Work out the finished part from the listing and answer in its coordinate system (mm). Round coordinates to 2 decimals unless told otherwise and drop trailing zeros. Order: outer loops, then holes, each group sorted by start corner. A loop starts at its lowest first (then second) coordinate and runs counter-clockwise, first axis right, second up. Notation, with made-up numbers: (24.5, 55) - (51.5, 55) arc R36 ccw to (51.5, 90) - close; hole circle Ø3 at (20, 75.25). An arc over 180 degrees is marked (long way). Use one line per item in the form item = value. Start each with the question number.
Q1. The part is cut by section D-D on x = 12.5. Determine the outline of the cut face in (y, z), plus the area to 3 significant figures.
Q2. The part is cut by section C-C on x = -74.5. Determine the outline of the cut face in (y, z), plus the area to 3 significant figures.
Q3. Given P1, Ø3, axis at y = -37.5, z = 2.5, coming from the +X side; P2, Ø6, axis at x = -55, z = 4.5, coming from the +Y side; P3, Ø2, axis at x = 41, z = 2.5, coming from the +Y side, each flat-ended and moving along its own axis, determine where each tip first touches the part or whether it passes through.
Q4. The part is cut by section A-A on z = 8.25. Determine the outline of the cut face in (x, y).
Q5. Find the intervals of material crossed by line 1 (X direction, y = 34, z = 1.25); line 2 (Y direction, x = 45.5, z = 9.75); line 3 (X direction, y = -78, z = 5.25), in increasing order. Write a range as [from, to].
Q6. The part is cut by section B-B on y = 0. Determine the outline of the cut face in (x, z).
from build123d import *

# Parameters (mm, degrees)
SKETCH2_R           = 40
BOSS_EXTRUDE1_DEPTH = 10


with BuildPart() as part:
    # Sketch2 → Boss-Extrude1 (new body)
    with BuildSketch(Plane.XY):
        with BuildLine():
            Line((-100, -40), (-100, -30))
            ThreePointArc((-100, -30), (-70, 0), (-100, 30))
            Line((-100, 30), (-100, 40))
            ThreePointArc((-100, 40), (-84.220237409, 36.755939555), (-71, 27.549954628))
            ThreePointArc((-71, 27.549954628), (-55.218260111, 21.366045629), (-40.357142857, 29.51780853))
            ThreePointArc((-40.357142857, 29.51780853), (-23.282031855, 44.248694813), (-1.47081146, 49.978362455))
            ThreePointArc((-1.47081146, 49.978362455), (15.390674553, 60.197087002), (15.293909304, 79.913138291))
            ThreePointArc((15.293909304, 79.913138291), (11.346128086, 89.510287366), (10, 99.8))
            Line((10, 99.8), (20, 99.8))
            ThreePointArc((20, 99.8), (50, 69.8), (80, 99.8))
            Line((80, 99.8), (90, 99.8))
            ThreePointArc((90, 99.8), (79.950139168, 73.286057181), (54.85054181, 60.095186134))
            ThreePointArc((54.85054181, 60.095186134), (39.000828287, 48.368352667), (40.911294797, 28.744842286))
            ThreePointArc((40.911294797, 28.744842286), (50, 0), (40.911294797, -28.744842286))
            ThreePointArc((40.911294797, -28.744842286), (39.000828287, -48.368352667), (54.85054181, -60.095186134))
            ThreePointArc((54.85054181, -60.095186134), (79.950139168, -73.286057181), (90, -99.8))
            Line((90, -99.8), (80, -99.8))
            ThreePointArc((80, -99.8), (50, -69.8), (20, -99.8))
            Line((20, -99.8), (10, -99.8))
            ThreePointArc((10, -99.8), (11.346128086, -89.510287366), (15.293909304, -79.913138291))
            ThreePointArc((15.293909304, -79.913138291), (15.390674553, -60.197087002), (-1.47081146, -49.978362455))
            ThreePointArc((-1.47081146, -49.978362455), (-23.282031855, -44.248694813), (-40.357142857, -29.51780853))
            ThreePointArc((-40.357142857, -29.51780853), (-55.218260111, -21.366045629), (-71, -27.549954628))
            ThreePointArc((-71, -27.549954628), (-84.220237409, -36.755939555), (-100, -40))
        make_face()
        Circle(SKETCH2_R, mode=Mode.SUBTRACT)
    extrude(amount=BOSS_EXTRUDE1_DEPTH)


solid = part.part
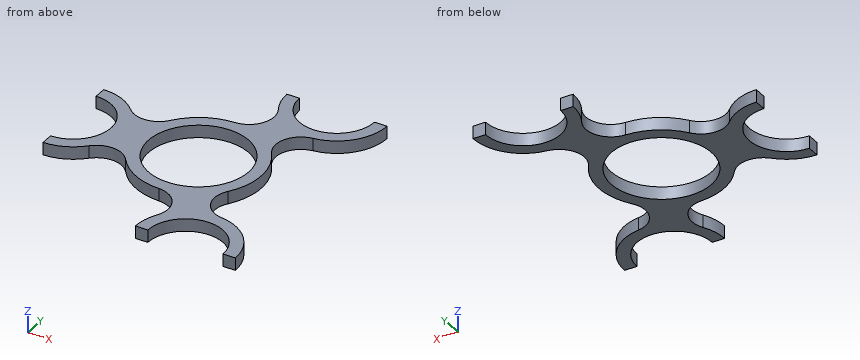
Found:
q1.outline = (-99.8, 0) - (-85.88, 0) - (-85.88, 10) - (-99.8, 10) - close; (-56.26, 0) - (-38, 0) - (-38, 10) - (-56.26, 10) - close; (38, 0) - (56.26, 0) - (56.26, 10) - (38, 10) - close; (85.88, 0) - (99.8, 0) - (99.8, 10) - (85.88, 10) - close
q1.area = 644 mm²
q2.outline = (-30.82, 0) - (-15.8, 0) - (-15.8, 10) - (-30.82, 10) - close; (15.8, 0) - (30.82, 0) - (30.82, 10) - (15.8, 10) - close
q2.area = 300 mm²
q3.P1 = 37.73
q3.P2 = 21.84
q3.P3 = 71.52
q4.outline = (-100, -40) arc R40 ccw to (-71, -27.55) arc R20 cw to (-40.36, -29.52) arc R50 ccw to (-1.47, -49.98) arc R20 cw to (15.29, -79.91) arc R40 ccw to (10, -99.8) - (20, -99.8) arc R30 cw to (80, -99.8) - (90, -99.8) arc R40 ccw to (54.85, -60.1) arc R20 cw to (40.91, -28.74) arc R50 ccw to (40.91, 28.74) arc R20 cw to (54.85, 60.1) arc R40 ccw to (90, 99.8) - (80, 99.8) arc R30 cw to (20, 99.8) - (10, 99.8) arc R40 ccw to (15.29, 79.91) arc R20 cw to (-1.47, 49.98) arc R50 ccw to (-40.36, 29.52) arc R20 cw to (-71, 27.55) arc R40 ccw to (-100, 40) - (-100, 30) arc R30 cw to (-100, -30) - close; hole circle Ø80 at (0, 0)
q5.line_1 = [-100, -78.93], [-36.66, -21.07], [21.07, 38.28]
q5.line_2 = [-70.14, -56.41], [-20.73, 20.73], [56.41, 70.14]
q5.line_3 = [16.26, 29.39], [70.61, 83.54]
q6.outline = (-70, 0) - (-40, 0) - (-40, 10) - (-70, 10) - close; (40, 0) - (50, 0) - (50, 10) - (40, 10) - close
